Can you work these out from the model? Positions are in its coordinate system, mm. A direction names the side the tool comes from. Give positions to 0.01 mm unless a question says otherwise; leave off trailing zeros. Write each loop counter-clockwise with the first axis right and the second up, starting at its lowest first coordinate (ties: lowest second). Pieces come first, ordered by that corner, then holes. Notation, with made-up numbers: M 3,56 L 11,56 A4 cw 11,60 Z; hole C 87,5.5 d5. An arc over 180 degrees is marked long. Write each question's results on one line, items separated by ' | '.
from build123d import *

# Parameters (mm, degrees)
SKETCH1_R                = 14.5
SKETCH1_R_2              = 10.5
BOSS_EXTRUDE1_DEPTH      = 20
SKETCH2_R                = 15.3
SKETCH2_R_2              = 11
BOSS_EXTRUDE2_DEPTH      = 19.5
DRAFT1_ANGLE             = 1
BOSS_EXTRUDE3_REACH      = 71.659
BOSS_EXTRUDE3_END_RADIUS = 14.5
SKETCH4_R                = 14.5
SKETCH5_R                = 15.35
BOSS_EXTRUDE4_DEPTH      = 19.5
SKETCH6_R                = 11
CUT_EXTRUDE1_DEPTH       = 40


# Read off the part's stored shape, not the designer's step: Mirror1
with BuildPart() as part:
    # Sketch1 → Boss-Extrude1 (new, symmetric)
    with BuildSketch(Plane.XY):
        Circle(SKETCH1_R)
        Circle(SKETCH1_R_2, mode=Mode.SUBTRACT)
    extrude(amount=BOSS_EXTRUDE1_DEPTH, both=True)

    # Sketch2 → Boss-Extrude2 (add)
    with BuildSketch(Plane.XY.offset(20)):
        Circle(SKETCH2_R)
        Circle(SKETCH2_R_2, mode=Mode.SUBTRACT)
    extrude(amount=BOSS_EXTRUDE2_DEPTH)

    # Draft1
    draft1_faces = [part.faces().sort_by_distance(p)[0] for p in [
        (-11, 0, 29.75),
    ]]
    draft(draft1_faces, Plane.XY.offset(20), DRAFT1_ANGLE)

    # Mirror1 outline → Mirror1 (revolve)
    with BuildSketch(Plane.XZ):
        Polygon((15.3, -39.5), (15.3, -20), (10.5, -20), (10.5, -8.644980815), (9.961423637, -39.5), align=None)
    revolve(axis=Axis((0, 0, 0), (0, 0, 1)))

    # Boss-Extrude3: up to this cylinder (the profile starts outside it)
    boss_extrude3_end = Plane(origin=(0, 0, 0), z_dir=(0, 0, -1)) * Cylinder(BOSS_EXTRUDE3_END_RADIUS, 173.318, mode=Mode.PRIVATE)
    # Sketch4 → Boss-Extrude3 (add, up to the surface)
    with BuildSketch(Plane(origin=(0, 40, 0), x_dir=(1, 0, 0), z_dir=(0, 1, 0)), mode=Mode.PRIVATE) as boss_extrude3_sk1:
        with Locations(Location((0, 0, 0), (0, 0, 270))):
            Circle(SKETCH4_R)
    boss_extrude3_tool1 = extrude(boss_extrude3_sk1.sketch, amount=-BOSS_EXTRUDE3_REACH, mode=Mode.PRIVATE) - boss_extrude3_end
    add(boss_extrude3_tool1.solids().sort_by_distance((0, 40, 0))[0])

    # Sketch5 → Boss-Extrude4 (add)
    with BuildSketch(Plane(origin=(0, 40, 0), x_dir=(1, 0, 0), z_dir=(0, 1, 0))):
        with Locations(Location((0, 0, 0), (0, 0, 270))):
            Circle(SKETCH5_R)
    extrude(amount=-BOSS_EXTRUDE4_DEPTH)

    # Sketch6 → Cut-Extrude1 (cut)
    with BuildSketch(Plane(origin=(0, 40, 0), x_dir=(1, 0, 0), z_dir=(0, 1, 0))):
        with Locations(Location((0, 0, 0), (0, 0, 270))):
            Circle(SKETCH6_R)
    extrude(amount=-CUT_EXTRUDE1_DEPTH, mode=Mode.SUBTRACT)


solid = part.part
Item 1: If I drill on line 1 (X direction, y = 0, z = 4); line 2 (X direction, y = 18, z = 0); line 3 (Y direction, x = 3, z = -11.5), over which ranges is the centre line in solid material (lowest first)? Write a range as from..to.
Geometry says:
line 1: x = -14.5..-10.5, 10.5..14.5 | line 2: x = -14.5..-11, 11..14.5 | line 3: y = -14.19..-10.01, 10.01..40
Item 2: I want a section at C-C, the plane x = -12.5. Please give me the cut outline in (y, z).
Geometry says:
outline: M -8.82,-39.5 L 8.82,-39.5 L 8.82,-20 L 7.35,-20 L 7.35,-7.35 L 20.5,-7.35 L 20.5,-8.91 L 40,-8.91 L 40,8.91 L 20.5,8.91 L 20.5,7.35 L 7.35,7.35 L 7.35,20 L 8.82,20 L 8.82,39.5 L -8.82,39.5 L -8.82,20 L -7.35,20 L -7.35,-20 L -8.82,-20 Z
Item 3: I'm going to push flat-ended pins straight in: pin 1 (2 mm diameter, centred on y = 4.5, z = -26, fed in from +X); pin 2 (12.5 mm diameter, centred on x = 0, y = 0, fed in from -Z); pin 3 (4 mm diameter, centred on x = 12, y = 22.5, fed in from -Z); pin 4 (10 mm diameter, centred on x = 5, z = -25.5, fed in from +Y). Where does each tip first touch, or does it pass through?
Geometry says:
pin 1: stops at x = 14.89 | pin 2: passes through | pin 3: stops at z = -11.65 | pin 4: stops at y = 15.3
Item 4: Thinking about a two-plate mould opening in Z: for faces 4 (the face through (3.304, 24.724, 10.492)), 5 (the face through (10.652, 3.355, 29.614)), 6 (the face through (12.4, -7.9, 20)), 7 (the face through (-7, 40, 10)), which applies, +Z half, -Z half, draft (parallel to the pull), parting line (faces both ways), or undercut?
Geometry says:
face 4: undercut | face 5: +Z half | face 6: undercut | face 7: draft
Item 5: I want a section at A-A, the plane z = 0. Please give me the cut outline in (x, y).
Geometry says:
outline: M -15.35,20.5 L -14.5,20.5 L -14.5,0 A14.5 ccw 14.5,0 L 14.5,20.5 L 15.35,20.5 L 15.35,40 L 11,40 L 11,0 L 10.5,0 A10.5 cw -10.5,0 L -11,0 L -11,40 L -15.35,40 Z
Item 6: I want a section at D-D, the plane z = -13.5. Please give me the cut outline in (x, y).
Geometry says:
outline: M -7.31,20.5 L -5.29,20.5 L -5.29,13.5 A14.5 ccw long 5.29,13.5 L 5.29,20.5 L 7.31,20.5 L 7.31,40 L -7.31,40 Z; hole C 0,0 d20.83
Item 7: I want a section at B-B, the plane y = 17. Please give me the cut outline in (x, z).
Geometry says:
outline: C 0,0 d29; hole C 0,0 d22
Item 8: For faces 1 (the face through (-9.34, 30.39, -12.18)), 2 (the face through (-2.217, -9.984, -24.288)), 3 (the face through (-3.143, -14.155, 0.28)), which set-ups out of +Z, -Z, +X, -X, +Y, -Y let a thin tool reach every point of the face, with its end or its side?
Geometry says:
face 1: +Y | face 2: +Z | face 3: none
